For this review, take the finished solid that the model builds, in its own axes (mm). A direction names the side the tool comes from. Round coordinates to 2 decimals unless told otherwise and drop trailing zeros. Write each question's results on one line, items separated by ' | '. Start each with the question number.
(1) For faces 4 (the flat face through (-323.85, 2, 6)), 5 (the flat face through (-1, 0, 6)), 6 (the flat face through (230, 107.95, 6)), list the 3-axis set-ups (+Z, -Z, +X, -X, +Y, -Y) from which the entire face can be reached by the end or side of a thin tool; tool diameter is ignored.
(2) Insertion check: pin 1 Ø6.5 at (y, z) = (166.5, 3.5) entering from +X; pin 2 Ø4 at (x, z) = (-208.5, 7) entering from +Y; pin 3 Ø5.5 at (x, y) = (-114.3, -53.77) entering from +Z. Each pin has a flat end and moves straight along its axis. Give the tip position at first contact, or say it passes through.
(3) Draft analysis for pull direction Y (two halves, no side actions). For faces 1 (the cylindrical face through (-18.583, 24.264, 5.478)), 2 (the flat face through (-26, 7, 12.7)), 3 (the flat face through (2, 215.9, 6)), state which applies: pulls with the +Y half, pulls with the -Y half, needs draft (parallel to the pull), parting line crosses it, or undercut.
(4) Take a section at B-B, the plane y = -18.5. Give the number of separate pieces and of enclosed holes in the cut face, plus the area to 3 significant figures.
(5) For L1, parallel to Y at x = -317.5, z = 7.5; L2, parallel to X at y = -90.5, z = 3, list the stretches that pass through material, from the lowest coordinate up. Write a range as from..to.
```python
from build123d import *

# Parameters (mm, degrees)
F0_R           = 85.725
F1_DEPTH       = 12.7
F3_D           = 4.7625
F3_CSINK_D     = 7.9375
F3_CSINK_ANGLE = 85
F4_SIZE        = 1.5875


# Not quite as in the source:
# - a feature names something its author has since deleted; it is built from what else it names


with BuildPart() as f1:
    # F0 (on Top) → F1 (new body)
    with BuildSketch(Plane.XY):
        Polygon((-107.95, 133.35), (-133.35, 107.95), (-323.85, 107.95), (-323.85, -107.95), (-107.95, -107.95), (-107.95, -25.4), (-82.55, 0), (82.55, 0), (107.95, -25.4), (107.95, -107.95), (323.85, -107.95), (323.85, 107.95), (133.35, 107.95), (107.95, 133.35), (107.95, 215.9), (-107.95, 215.9), align=None)
        with Locations((-215.9, 0)):
            Circle(F0_R, mode=Mode.SUBTRACT)
        with Locations((215.9, 0)):
            Circle(F0_R, mode=Mode.SUBTRACT)
        with Locations((0, 107.95)):
            Circle(F0_R, mode=Mode.SUBTRACT)
    extrude(amount=F1_DEPTH)

    # F3 (through all)
    with Locations(Plane.XY.offset(12.7)):
        with Locations((-239.6099832965, 101.6), (-161.7199665929, 101.6), (-116.1598719395, 116.1598719395), (-101.6, 161.7199665929), (-101.6, 209.55), (-33.8666666667, 209.55), (33.8666666667, 209.55), (101.6, 209.55), (101.6, 161.7199665929), (116.1598719395, 116.1598719395), (161.7199665929, 101.6), (239.6099832965, 101.6), (317.5, 33.8666666667), (317.5, 101.6), (317.5, -33.8666666667), (317.5, -101.6), (249.7666666667, -101.6), (182.0333333333, -101.6), (114.3, -53.7699665929), (114.3, -101.6), (99.7401280605, -8.2098719395), (54.1800334071, 6.35), (0, 6.35), (-54.1800334071, 6.35), (-99.7401280605, -8.2098719395), (-114.3, -53.7699665929), (-114.3, -101.6), (-182.0333333333, -101.6), (-249.7666666667, -101.6), (-317.5, -101.6), (-317.5, -33.8666666667), (-317.5, 33.8666666667), (-317.5, 101.6)):
            CounterSinkHole(F3_D / 2, F3_CSINK_D / 2, counter_sink_angle=F3_CSINK_ANGLE)

    # F4
    f4_edges = [f1.edges().sort_by_distance(p)[0] for p in [
        (-85.725, 107.95, 12.7),
        (-301.625, 0, 12.7),
        (130.175, 0, 12.7),
    ]]
    chamfer(f4_edges, length=F4_SIZE)


solid = f1.part
```
Results below:
1) face 4: +Z, -Z, -X, +Y, -Y | face 5: +Z, -Z, -Y | face 6: +Z, -Z, +X, +Y
2) pin 1: stops at x = 107.95 | pin 2: stops at y = 107.95 | pin 3: stops at z = 11.37
3) face 1: undercut | face 2: needs draft | face 3: pulls with the +Y half
4) separate pieces: 4 | enclosed holes: 0 | area: 1,400 mm^2
5) L1: y = -107.95..-103.98, -99.22..-36.25, -31.49..31.49, 36.25..99.22, 103.98..107.95 | L2: x = -323.85..-107.95, 107.95..323.85
